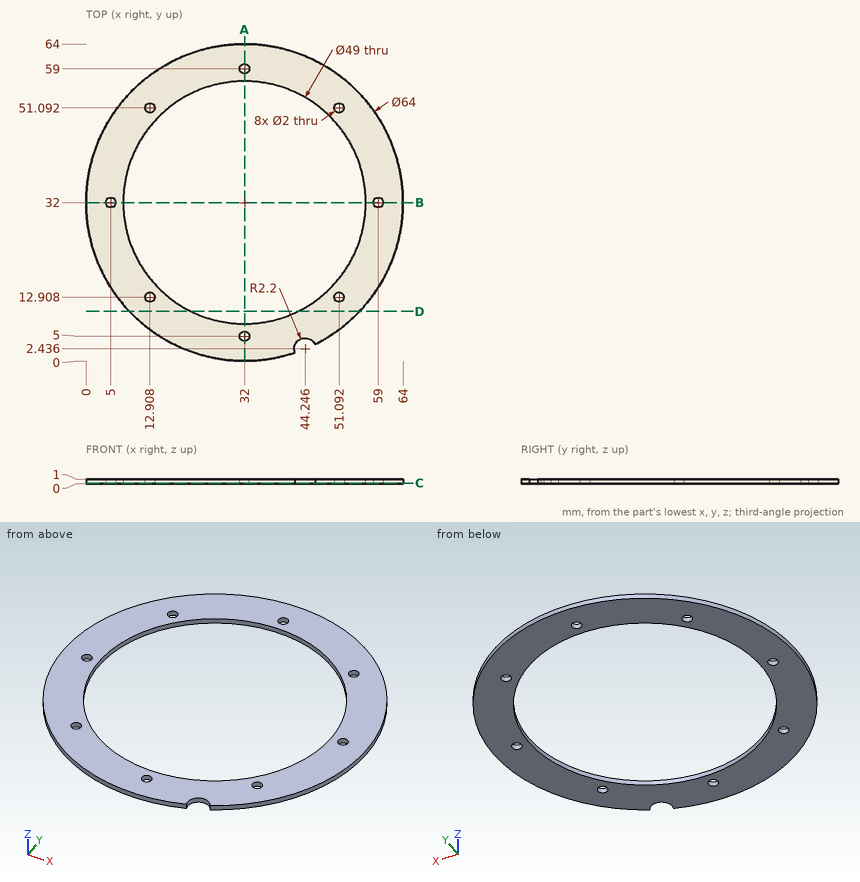
Answer from the drawing. Dimensions are ordinates in mm from the lowest x, y and z of the part. Round coordinates to 2 decimals unless told otherwise and drop trailing zeros. Order: outer loops, then holes, each group sorted by start corner. A loop starts at its lowest first (then second) coordinate and runs counter-clockwise, first axis right, second up. Notation, with made-up numbers: (65.25, 64.25) - (77.25, 64.25) arc R18 ccw to (77.25, 94.25) - close; hole circle Ø11 at (25.5, 27.25). An arc over 180 degrees is marked (long way). Put each result on its own line as item: value. Start each with the question number.
(1) Find section A-A (x = 32). Give the vertices of the cut face in (y, z).
(2) Straight lines are drawn through the part: probe 1 along Y at (x, z) = (32, 0.5); probe 2 along X at (y, z) = (13.5, 0.9) (1 decimal). For each, find the intervals that lie inside material, in ascending order. Write a range as from..to.
(3) Given P1, Ø2.5, axis at x = 32, y = 5, coming from the -Z side, flat-ended and moving along its own axis, determine where the tip first touches the part or whether it passes through.
(4) Find section C-C (z = 0.15). State how many separate pieces and enclosed holes the cut face has, plus the area to 3 significant figures.
(5) Find section D-D (y = 10). Give the vertices of the cut face in (x, z), plus the area to 3 significant figures.
Reply:
1. outline: (0, 0) - (4, 0) - (4, 1) - (0, 1) - close; (6, 0) - (7.5, 0) - (7.5, 1) - (6, 1) - close; (56.5, 0) - (58, 0) - (58, 1) - (56.5, 1) - close; (60, 0) - (64, 0) - (64, 1) - (60, 1) - close
2. probe 1: 0..4, 6..7.5, 56.5..58, 60..64
2. probe 2: 5.9..12.1, 13.7..15.9, 48.1..50.3, 51.9..58.1
3. P1: z = 0
4. separate pieces: 1
4. enclosed holes: 9
4. area: 1,300 mm^2
5. outline: (8.76, 0) - (21.22, 0) - (21.22, 1) - (8.76, 1) - close; (42.78, 0) - (55.24, 0) - (55.24, 1) - (42.78, 1) - close
5. area: 24.9 mm^2
